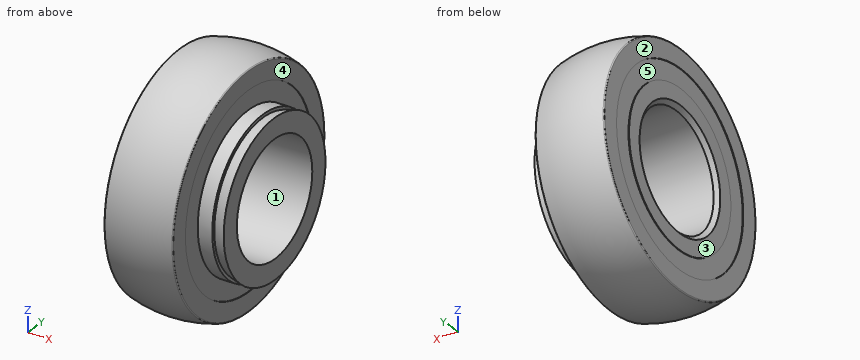
Solid Edge part; units mm, degrees
sketch "Sketch1" plane through (0, 0, 0) normal (0, 0, 1) x (1, 0, 0)
  line L0 (-6, 19.975) -> (-6, 16.8)
  line L1 (-6, 16.8) -> (-5.9, 16.8)
  line L2 (-5.9, 16.8) -> (-5.9, 13.5)
  line L3 (-5.9, 13.5) -> (-6, 13.5)
  line L4 (-6, 13.5) -> (-6, 10.7071)
  line L5 (-6, 10.7071) -> (-5.2929, 10)
  line L6 (-5.2929, 10) -> (10.5, 10)
  line L7 (10.5, 10) -> (10.5, 13.5)
  line L8 (10.5, 13.5) -> (8.5, 12.9641)
  line L9 (8.5, 12.9641) -> (8.5, 13.5)
  line L10 (8.5, 13.5) -> (6, 13.5)
  line L11 (6, 13.5) -> (6, 13.4)
  line L12 (6, 13.4) -> (5.9, 13.4)
  line L13 (5.9, 13.4) -> (5.9, 16.8)
  line L14 (5.9, 16.8) -> (6, 16.8)
  line L15 (6, 16.8) -> (6, 19.975)
  arc A0 (6, 19.975) -> (5.8558, 20.1671) centre (5.8, 19.975) ccw
  arc A1 (5.8558, 20.1671) -> (-5.8558, 20.1671) centre (0, 0) ccw
  arc A2 (-5.8558, 20.1671) -> (-6, 19.975) centre (-5.8, 19.975) ccw
revolve "RevolvedProtrusion1" add sketch "Sketch1" angle 360 about axis through (10.5, 0, 0) along (-1, 0, 0)
properties part number "62599720_2"
Part model, mm, in its own coordinate system. Face numbers are marked on the shaded views. A direction names the side the tool comes from. Give positions to 0.01 mm unless a question says otherwise; leave off trailing zeros. Loops run counter-clockwise (first coordinate to the right, second up) from the corner with the lowest first, then second, coordinate; pieces in that order, holes last.
(1) Band-saw the part on A-A (x = 0). Write the cut outline in (y, z).
Return value:
outline: circle Ø42 at (0, 0); hole circle Ø20 at (0, 0)
(2) Pull direction Y, two halves, no side cores. Call the marked faces 1 and 2: pulls with the +Y half, pulls with the -Y half, needs draft (parallel to the pull), parting line crosses it, or undercut.
Return value:
face 1: undercut
face 2: needs draft
(3) Band-saw the part on B-B (x = 7.25). Write the cut outline in (y, z), and give its area (3 significant figures).
Return value:
outline: circle Ø27 at (0, 0); hole circle Ø20 at (0, 0)
area: 258 mm2
(4) Pin check, flat tips, straight feed: pin 1 (4 mm diameter, centred on x = -2.5, z = -14.5, fed in from -Y); pin 2 (8 mm diameter, centred on x = 0, z = -13.5, fed in from +Y); pin 3 (1.5 mm diameter, centred on y = 7.5, z = -2.5, fed in from -X); pin 4 (1 mm diameter, centred on x = 0.5, z = -4.5, fed in from -Y). Stop position of each tip, or through.
Return value:
pin 1: stops at y = -16.71
pin 2: stops at y = 18.73
pin 3: passes through
pin 4: stops at y = -20.61
(5) 3-axis set-ups, long thin cutter, end or side, ignore diameter. For the marked faces 3, 4 and 5: which of +Z, -Z, +X, -X, +Y, -Y reach the whole face in a straight line?
Return value:
face 3: +Z, -Z, -X, +Y, -Y
face 4: +X
face 5: -X
(6) Drill centre lines: line 1 along X through (y, z) = (-16.5, 2); line 2 along Y through (x, z) = (6.75, -5); line 3 along Y through (x, z) = (-5.85, 0). Where is each one in solid material? Low to high.
Return value:
line 1: x = -5.9 to 5.9
line 2: y = -12.54 to -8.66, 8.66 to 12.54
line 3: y = -20.17 to -10.56, 10.56 to 20.17
